Model file for the job. Use its own axes, mm. Face numbers are marked on the shaded views. A direction names the side the tool comes from. Coordinates: 2 decimals unless noted, no trailing zeros. Write each loop counter-clockwise with the first axis right and the second up, starting at its lowest first coordinate (ties: lowest second). Pieces come first, ordered by that corner, then holes. Notation, with made-up numbers: (-1.5, 44) -> (35.5, 44) arc R8 cw to (35.5, 50) -> close; hole circle Ø3 at (55.5, 18). An arc over 180 degrees is marked (long way). Answer as a JSON object with one key per item and string values. Group by question number.
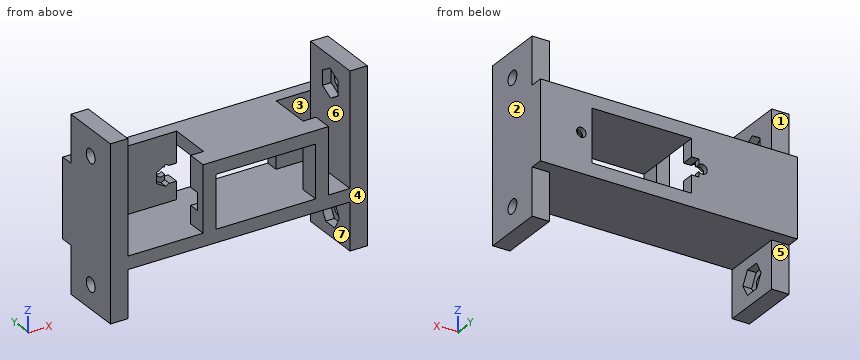
from build123d import *

# Parameters (mm, degrees)
BOSS_EXTRUDE1_DEPTH      = 3
SKETCH2_W                = 5
SKETCH2_H                = 3
SKETCH2_W_2              = 3
SKETCH2_H_2              = 4.533238731
BOSS_EXTRUDE2_DEPTH      = 15.2
BOSS_EXTRUDE3_DEPTH      = 3
BOSS_EXTRUDE4_DEPTH      = 19.425
BOSS_EXTRUDE5_DEPTH      = 6.955
CUT_EXTRUDE1_REACH       = 19.35
SKETCH6_R                = 1.1
CUT_EXTRUDE2_DEPTH       = 1.7
SKETCH8_W                = 4
SKETCH8_H                = 14.35
BOSS_EXTRUDE6_DEPTH      = 26.1
BOSS_EXTRUDE6_DEPTH_BACK = 13.9
SKETCH10_R               = 1.6
CUT_EXTRUDE3_DEPTH       = 56.38
CUT_EXTRUDE3_DEPTH_BACK  = 5
CUT_EXTRUDE5_START       = -2
CUT_EXTRUDE5_DEPTH       = 55.38
CUT_EXTRUDE6_DEPTH       = 7.5
CUT_EXTRUDE6_DEPTH_BACK  = 15.316761
CUT_EXTRUDE7_REACH       = 24.725
SKETCH13_W               = 4
SKETCH13_H               = 2.5


with BuildPart() as part:
    # Sketch1 → Boss-Extrude1 (new body)
    with BuildSketch(Plane.XY):
        Polygon((16.5, 0), (16.5, -3), (11.5, -3), (11.5, -12.816761269), (14.5, -12.816761269), (14.5, -17.35), (-14.5, -17.35), (-14.5, -12.816761269), (-11.5, -12.816761269), (-11.5, -3), (-16.5, -3), (-16.5, 0), align=None)
    extrude(amount=BOSS_EXTRUDE1_DEPTH)

    # Sketch2 → Boss-Extrude2 (add)
    with BuildSketch(Plane(origin=(0, 0, 0), x_dir=(-1, 0, 0), z_dir=(0, 0, -1))):
        with Locations((-14, -1.5)):
            Rectangle(SKETCH2_W, SKETCH2_H)
        with Locations((14, -1.5)):
            Rectangle(SKETCH2_W, SKETCH2_H)
        with Locations((-13, -15.083380635)):
            Rectangle(SKETCH2_W_2, SKETCH2_H_2)
        with Locations((13, -15.083380635)):
            Rectangle(SKETCH2_W_2, SKETCH2_H_2)
    extrude(amount=BOSS_EXTRUDE2_DEPTH)

    # Sketch3 → Boss-Extrude3 (add)
    with BuildSketch(Plane(origin=(0, 0, -12.2), x_dir=(-1, 0, 0), z_dir=(0, 0, -1))):
        Polygon((-11.5, -17.35), (16.5, -17.35), (16.5, 0), (-16.5, 0), (-16.5, -17.35), align=None)
    extrude(amount=BOSS_EXTRUDE3_DEPTH)

    # Sketch4 → Boss-Extrude4 (add)
    with BuildSketch(Plane.ZY.offset(16.5)):
        Polygon((-15.2, -17.35), (-12.2, -17.35), (-12.2, -3), (3, -3), (3, 0), (-15.2, 0), align=None)
    extrude(amount=BOSS_EXTRUDE4_DEPTH)

    # Sketch5 → Boss-Extrude5 (add)
    with BuildSketch(Plane(origin=(16.5, 0, 0), x_dir=(0, 0, -1), z_dir=(1, 0, 0))):
        Polygon((-3, 0), (15.2, 0), (15.2, -17.35), (12.2, -17.35), (12.2, -3), (-3, -3), align=None)
    extrude(amount=BOSS_EXTRUDE5_DEPTH)

    # Sketch6 → Cut-Extrude1 (cut, up to next)
    with BuildSketch(Plane(origin=(0, 0, 0), x_dir=(1, 0, 0), z_dir=(0, 1, 0)), mode=Mode.PRIVATE) as cut_extrude1_sk1:
        with Locations((14, 6.1)):
            Circle(SKETCH6_R)
    cut_extrude1_tool1 = extrude(cut_extrude1_sk1.sketch, amount=-CUT_EXTRUDE1_REACH, mode=Mode.PRIVATE) & part.part
    add(cut_extrude1_tool1.solids().sort_by_distance((14, 0, -6.1))[0], mode=Mode.SUBTRACT)
    # Sketch6 → Cut-Extrude1 (cut, up to next)
    with BuildSketch(Plane(origin=(0, 0, 0), x_dir=(1, 0, 0), z_dir=(0, 1, 0)), mode=Mode.PRIVATE) as cut_extrude1_sk2:
        with Locations((-14, 6.1)):
            Circle(SKETCH6_R)
    cut_extrude1_tool2 = extrude(cut_extrude1_sk2.sketch, amount=-CUT_EXTRUDE1_REACH, mode=Mode.PRIVATE) & part.part
    add(cut_extrude1_tool2.solids().sort_by_distance((-14, 0, -6.1))[0], mode=Mode.SUBTRACT)

    # Sketch7 → Cut-Extrude2 (cut)
    with BuildSketch(Plane.XZ.offset(3)):
        Polygon((14, -3.675128869), (11.9, -4.887564435), (11.9, -7.312435565), (14, -8.524871131), (16.1, -7.312435565), (16.1, -4.887564435), align=None)
        Polygon((-14, -3.675128869), (-16.1, -4.887564435), (-16.1, -7.312435565), (-14, -8.524871131), (-11.9, -7.312435565), (-11.9, -4.887564435), align=None)
    extrude(amount=-CUT_EXTRUDE2_DEPTH, mode=Mode.SUBTRACT)

    # Sketch8 → Boss-Extrude6 (add, two sides)
    with BuildSketch(Plane.XY.offset(-12.2)) as boss_extrude6_sk:
        with Locations((-33.925, -10.175)):
            Rectangle(SKETCH8_W, SKETCH8_H)
        with Locations((21.455, -10.175)):
            Rectangle(SKETCH8_W, SKETCH8_H)
    extrude(amount=BOSS_EXTRUDE6_DEPTH)
    extrude(boss_extrude6_sk.sketch, amount=-BOSS_EXTRUDE6_DEPTH_BACK)

    # Sketch10 → Cut-Extrude3 (cut, two sides)
    with BuildSketch(Plane(origin=(-31.925, 0, 0), x_dir=(0, 0, -1), z_dir=(1, 0, 0))) as cut_extrude3_sk:
        with Locations((-7.9, -10.175)):
            Circle(SKETCH10_R)
        with Locations((20.65, -10.175)):
            Circle(SKETCH10_R)
    extrude(amount=CUT_EXTRUDE3_DEPTH, mode=Mode.SUBTRACT)
    extrude(cut_extrude3_sk.sketch, amount=-CUT_EXTRUDE3_DEPTH_BACK, mode=Mode.SUBTRACT)

    # Sketch11 → Cut-Extrude5 (cut)
    with BuildSketch(Plane(origin=(-31.925, 0, 0), x_dir=(0, 0, -1), z_dir=(1, 0, 0)).offset(CUT_EXTRUDE5_START)):
        Polygon((-9.652389588, -12.960521627), (-6.363862302, -13.085374714), (-4.611472715, -10.299853087), (-6.147610412, -7.389478373), (-9.436137698, -7.264625286), (-11.188527285, -10.050146913), align=None)
        Polygon((20.65, -13.465896534), (23.5, -11.820448267), (23.5, -8.529551733), (20.65, -6.884103466), (17.8, -8.529551733), (17.8, -11.820448267), align=None)
    extrude(amount=CUT_EXTRUDE5_DEPTH, mode=Mode.SUBTRACT)

    # Sketch12 → Cut-Extrude6 (cut, two sides)
    with BuildSketch(Plane(origin=(0, 0, 0), x_dir=(1, 0, 0), z_dir=(0, 1, 0))) as cut_extrude6_sk:
        Polygon((-11.5, 6.1), (-11.5, 4.1), (-13.2, 4.1), (-13.2, 8.1), (-11.5, 8.1), align=None)
    extrude(amount=CUT_EXTRUDE6_DEPTH, mode=Mode.SUBTRACT)
    extrude(cut_extrude6_sk.sketch, amount=-CUT_EXTRUDE6_DEPTH_BACK, mode=Mode.SUBTRACT)

    # Sketch13 → Cut-Extrude7 (cut, up to next)
    with BuildSketch(Plane(origin=(-13.2, 0, 0), x_dir=(0, 0, -1), z_dir=(1, 0, 0)), mode=Mode.PRIVATE) as cut_extrude7_sk1:
        with Locations((6.1, -14.066761269)):
            Rectangle(SKETCH13_W, SKETCH13_H)
    cut_extrude7_tool1 = extrude(cut_extrude7_sk1.sketch, amount=-CUT_EXTRUDE7_REACH, mode=Mode.PRIVATE) & part.part
    add(cut_extrude7_tool1.solids().sort_by_distance((-13.2, -14.066761, -6.1))[0], mode=Mode.SUBTRACT)


solid = part.part
(1) Cut at C-C on z = 4. List the corners of the cut face in (x, y) (3 decimals).
(2) Pull direction Y, two halves, no side cores. Call the marked faces 1, 2, 3 and 4: released by +Y, released by -Y, zero draft, split by the parting line, or undercut.
(3) Pin check, flat tips, straight feed: pin 1 (2 mm diameter, centred on x = -9, y = -14, fed in from +Z); pin 2 (0.5 mm diameter, centred on x = -12, z = -6, fed in from +Y); pin 3 (5 mm diameter, centred on x = -17.5, z = -5.5, fed in from -Y). Stop position of each tip, or through.
(4) Cut at B-B on x = -9.5. List the corners of the cut face in (y, z).
(5) Wall check: probe 1 along X at (y, z) = (-4.5, 1) (3 decimals); probe 2 along X at (y, z) = (-2.5, -5.5) (3 decimals); probe 3 along X at (y, z) = (-11, -16) (3 decimals). Give the ranges that are in metal, low to high.
(6) Cut at D-D on z = -6.1. Give the number of separate pieces and of enclosed holes in the cut face, plus the area to 3 significant figures.
(7) 3-axis set-ups, long thin cutter, end or side, ignore diameter. For the marked faces 5, 6 and 7: which of +Z, -Z, +X, -X, +Y, -Y reach the whole face in a straight line?
(8) Cut at A-A on y = -4. List the corners of the cut face in (x, z) (3 decimals), plus the area to 3 significant figures.
Results found:
{
 "1": {"outline": "(-35.925, -17.35) -> (-31.925, -17.35) -> (-31.925, -3) -> (-35.925, -3) -> close; (19.455, -17.35) -> (23.455, -17.35) -> (23.455, -3) -> (19.455, -3) -> close"},
 "2": {"face 1": "released by +Y", "face 2": "zero draft", "face 3": "undercut", "face 4": "released by -Y"},
 "3": {"pin 1": "stops at z = 3", "pin 2": "stops at y = -15.32", "pin 3": "stops at y = -3"},
 "4": {"outline": "(-17.35, -15.2) -> (0, -15.2) -> (0, -12.2) -> (-17.35, -12.2) -> close; (-17.35, 0) -> (0, 0) -> (0, 3) -> (-17.35, 3) -> close"},
 "5": {"probe 1": "x = -35.925 to -31.925, -11.5 to 11.5, 19.455 to 23.455", "probe 2": "x = -35.925 to -16.1, 11.5 to 11.9, 16.1 to 23.455", "probe 3": "x = -35.925 to -31.925, 19.455 to 23.455"},
 "6": {"separate pieces": "5", "enclosed holes": "0", "area": "221 mm²"},
 "7": {"face 5": "-Z, +X, -X, +Y", "face 6": "+Z, -Y", "face 7": "-Z, +Y, -Y"},
 "8": {"outline": "(-35.925, -26.1) -> (-31.925, -26.1) -> (-31.925, -15.2) -> (19.455, -15.2) -> (19.455, -26.1) -> (23.455, -26.1) -> (23.455, 13.9) -> (19.455, 13.9) -> (19.455, -12.2) -> (-31.925, -12.2) -> (-31.925, 13.9) -> (-35.925, 13.9) -> close; (-11.5, 0) -> (11.5, 0) -> (11.5, 3) -> (-11.5, 3) -> close", "area": "543 mm²"}
}
